Geometry check sheet. Reference: drawing and pictorial views, mm from the part's lowest x, y, z. A direction names the side the tool comes from. Round coordinates to 2 decimals unless told otherwise and drop trailing zeros. Order: outer loops, then holes, each group sorted by start corner. A loop starts at its lowest first (then second) coordinate and runs counter-clockwise, first axis right, second up.
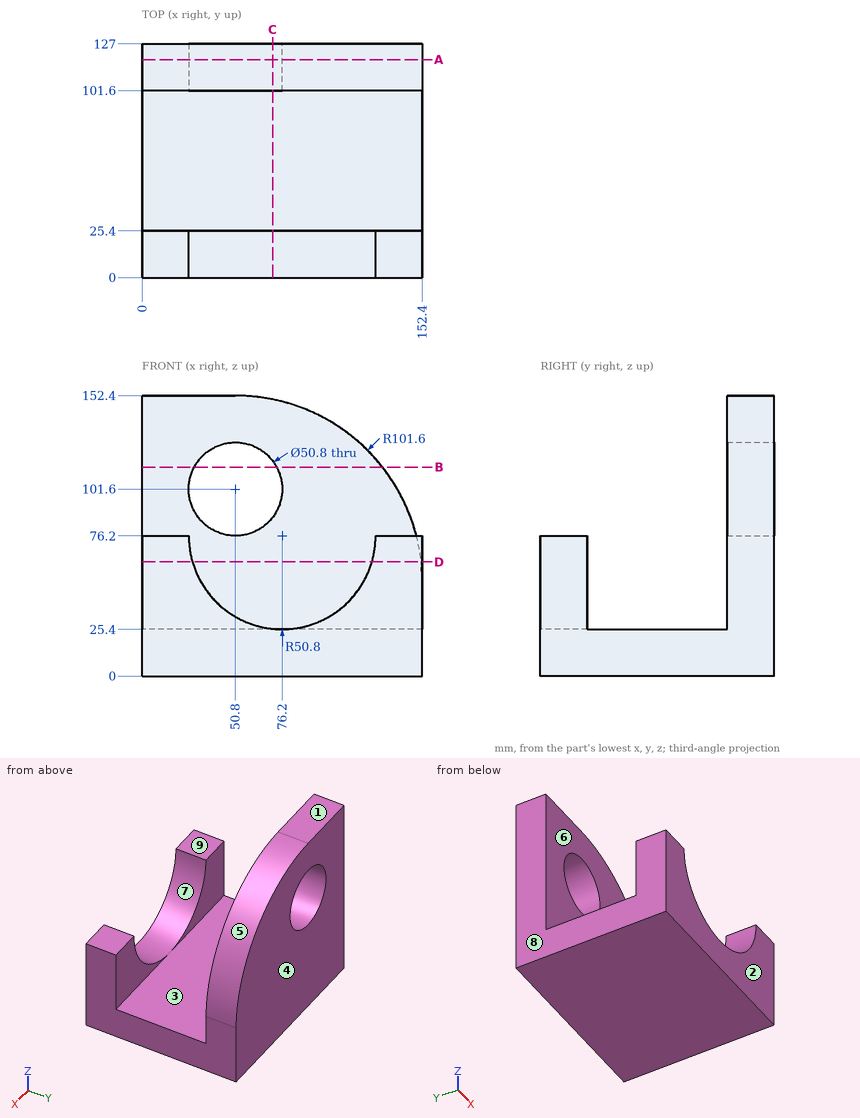
1) Sectioned sample at D-D on z = 62. Record the cut outline in (x, y) (3 decimals), then the cut area to 3 significant figures.
2) Go/stop test with flat-tipped pins: pin 1 Ø5 at (x, y) = (67.5, 102) entering from +Z; pin 2 Ø5 at (x, y) = (31, 87) entering from +Z; pin 3 Ø20.5 at (x, y) = (17.5, 15) entering from +Z. Record where each tip stops, or that it passes through.
3) Sectioned sample at B-B on z = 113.5. Record the cut outline in (x, y), then the cut area to 3 significant figures.
4) Sectioned sample at A-A on y = 118.5. Record the cut outline in (x, z).
5) Sectioned sample at C-C on x = 71. Record the cut outline in (y, z).
6) Draft check along Y on the marked faces 1, 2, 3 and 4. Enter one of: released by +Y, released by -Y, zero draft, split by the parting line, or undercut.
7) Scan lines: probe 1 along Z at (x, y) = (98, 71); probe 2 along Y at (x, z) = (88.5, 100); probe 3 along Z at (x, y) = (136.5, 5). Record each from-to range of solid material in increasing order.
8) Tool access check on the marked faces 5, 6, 7, 8 and 9. Record the directions out of +Z, -Z, +X, -X, +Y, -Y that give a thin tool (end or side, any length) a straight path to the whole face; none if there is none.
Returned:
1. outline: (0, 0) - (27.425, 0) - (27.425, 25.4) - (0, 25.4) - close; (0, 101.6) - (151.781, 101.6) - (151.781, 127) - (0, 127) - close; (124.975, 0) - (152.4, 0) - (152.4, 25.4) - (124.975, 25.4) - close
1. area: 5,250 mm2
2. pin 1: stops at z = 151.4
2. pin 2: stops at z = 25.4
2. pin 3: stops at z = 76.2
3. outline: (0, 101.6) - (28.36, 101.6) - (28.36, 127) - (0, 127) - close; (73.24, 101.6) - (130.75, 101.6) - (130.75, 127) - (73.24, 127) - close
3. area: 2,180 mm2
4. outline: (0, 0) - (152.4, 0) - (152.4, 50.8) arc R101.6 ccw to (50.8, 152.4) - (0, 152.4) - close; hole circle Ø50.8 at (50.8, 101.6)
5. outline: (0, 0) - (127, 0) - (127, 86.2) - (101.6, 86.2) - (101.6, 25.4) - (25.4, 25.4) - (25.4, 25.67) - (0, 25.67) - close; (101.6, 117) - (127, 117) - (127, 150.37) - (101.6, 150.37) - close
6. face 1: zero draft
6. face 2: released by -Y
6. face 3: undercut
6. face 4: released by +Y
7. probe 1: z = 0 to 25.4
7. probe 2: y = 101.6 to 127
7. probe 3: z = 0 to 76.2
8. face 5: +Z, +X, +Y
8. face 6: +Z, +X, -X
8. face 7: +Z, -Y
8. face 8: +Z, -Z, -X, +Y, -Y
8. face 9: +Z, +X, -X, -Y
